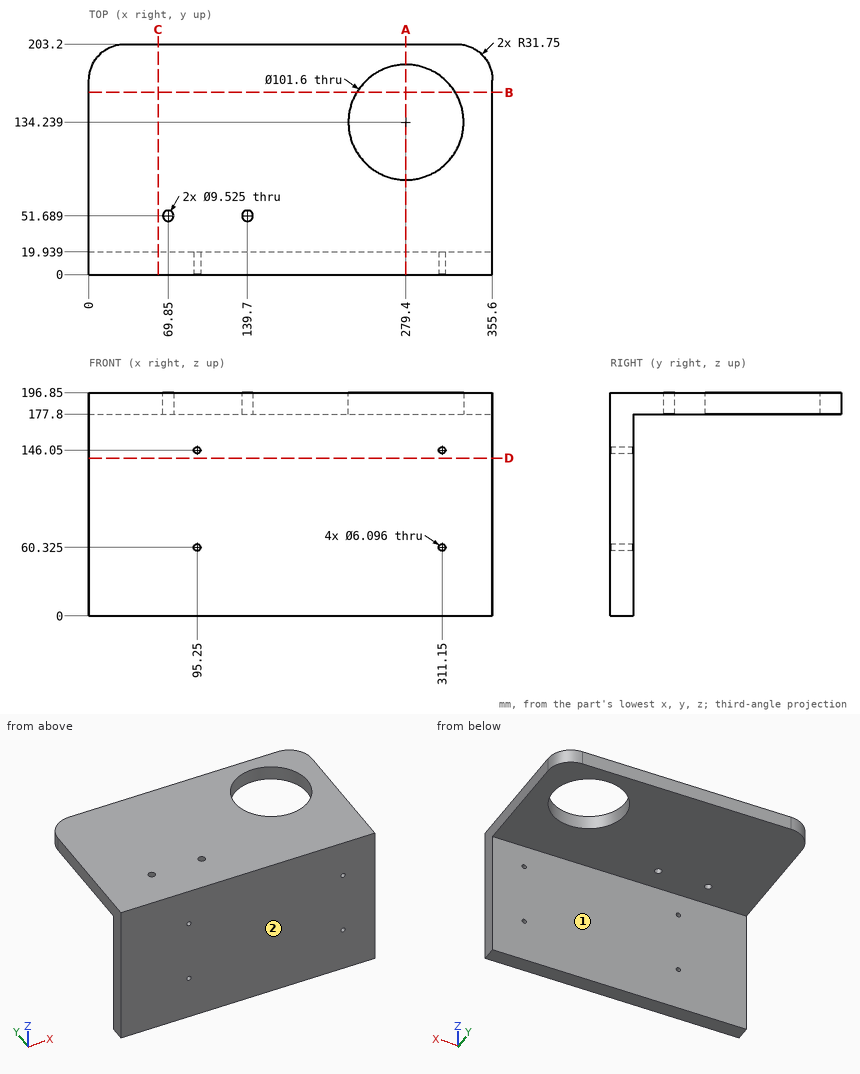
Part print with two shaded views. Sizes in mm from the minimum x, y, z corner. A direction names the side the tool comes from. Coordinates: 2 decimals unless noted, no trailing zeros. Order: outer loops, then holes, each group sorted by start corner. A loop starts at its lowest first (then second) coordinate and runs counter-clockwise, first axis right, second up. Notation, with made-up numbers: (77, 23.25) - (85, 23.25) arc R15 ccw to (85, 35.25) - close; hole circle Ø8 at (-16, 54). An arc over 180 degrees is marked (long way). Write item = value, one per line. Start each with the question number.
1) Saw through at D-D on z = 139. Write the cut outline in (x, y), then the cut area to 3 significant figures.
2) Saw through at B-B on y = 160.5. Write the cut outline in (x, z).
3) 3-axis set-ups, long thin cutter, end or side, ignore diameter. For the marked faces 1 and 2: which of +Z, -Z, +X, -X, +Y, -Y reach the whole face in a straight line?
4) Saw through at A-A on x = 279.4. Write the cut outline in (y, z), then the cut area to 3 significant figures.
5) Saw through at C-C on x = 61. Write the cut outline in (y, z), then the cut area to 3 significant figures.
6) Flat gauge pins, fed straight in: pin 1 Ø3 at (x, z) = (316, 50) entering from +Y; pin 2 Ø3 at (x, y) = (178, 177.5) entering from -Z. Where does each tip first touch, or does it go through?
7) Wall check: line 1 along X through (y, z) = (14.25, 146.05); line 2 along Y through (x, z) = (80, 20.5); line 3 along Y through (x, z) = (317, 185). Give the ranges that are in metal, low to high. Write a range as from..to.
From the geometry:
q1.outline = (0, 0) - (355.6, 0) - (355.6, 19.94) - (0, 19.94) - close
q1.area = 7,090 mm^2
q2.outline = (0, 177.8) - (235.91, 177.8) - (235.91, 196.85) - (0, 196.85) - close; (322.89, 177.8) - (355.6, 177.8) - (355.6, 196.85) - (322.89, 196.85) - close
q3.face_1 = -Z, +X, -X, +Y
q3.face_2 = +Z, -Z, +X, -X, -Y
q4.outline = (0, 0) - (19.94, 0) - (19.94, 177.8) - (83.44, 177.8) - (83.44, 196.85) - (0, 196.85) - close; (185.04, 177.8) - (203.2, 177.8) - (203.2, 196.85) - (185.04, 196.85) - close
q4.area = 5,480 mm^2
q5.outline = (0, 0) - (19.94, 0) - (19.94, 177.8) - (203.2, 177.8) - (203.2, 196.85) - (0, 196.85) - close
q5.area = 7,420 mm^2
q6.pin_1 = 19.94
q6.pin_2 = 177.8
q7.line_1 = 0..92.2, 98.3..308.1, 314.2..355.6
q7.line_2 = 0..19.94
q7.line_3 = 0..100.08, 168.4..203.2
